Autodesk Inventor part; units mm, degrees
ref_plane "YZ Plane" through (0, 0, 0) normal (1, 0, 0) x (0, 1, 0)
ref_plane "XZ Plane" through (0, 0, 0) normal (0, 1, 0) x (-1, 0, 0)
ref_plane "XY Plane" through (0, 0, 0) normal (0, 0, 1) x (1, 0, 0)
sketch "Sketch1" plane through (0, 0, 0) normal (0, 1, 0) x (-1, 0, 0)
  circle A0 centre (0, 0) radius 9.525
  dimension "d0" = 19.05
extrude "Extrusion1" add sketch "Sketch1" along normal blind 5
sketch "Sketch2" plane through (0, 5, 0) normal (0, 1, 0) x (1, 0, 0)
  line L0 (0, 0) -> (0, 6.5)
  point P0 (-6.5, 0)
  point P1 (0, -6.5)
  point P2 (6.5, 0)
  dimension "d3" = 6.5
  dimension "d6" = 360
hole "Hole1" at (0, 5, -6.5) at (0, 5, 6.5) at (-6.5, 5, 0) at (6.5, 5, 0) direction (0, -1, 0) diameter 2.459 end through all
sketch "Sketch3" plane through (0, 5, 0) normal (0, 1, 0) x (1, 0, 0)
  circle A0 centre (0, 0) radius 2.1
  dimension "d15" = 4.2
extrude "Extrusion2" cut sketch "Sketch3" against normal through all
chamfer "Chamfer1" distance 0.25 angle 45 4 edges at (-2.1, 5, 0) (9.525, 5, 0) (9.525, 0, 0) (-2.1, 0, 0)
move or copy body "Move Body1" bodies to move or copy 1 copy no rotation origin (0, 0, 0) rotation axis (0, 1, 0) rotation angle 45
sketch "Sketch4" plane through (0, 0, 0) normal (1, 0, 0) x (0, 1, 0)
  line L0 (0, 0) -> (2.5, 0)
  dimension "d22" = 2.5
hole "Hole2" at (0, 2.5, 0) direction (1, 0, 0) diameter 2.459 end through all
properties part number "pololu-mounting-hub"
Build history of the part. All positions in model axes, mm. Round coordinates to 2 decimals unless told otherwise and drop trailing zeros. Order: outer loops, then holes, each group sorted by start corner. A loop starts at its lowest first (then second) coordinate and runs counter-clockwise, first axis right, second up. Notation, with made-up numbers: (-4.5, -15.75) -> (12.5, -15.75) arc R31 ccw to (12.5, 17.25) -> close; hole circle Ø11 at (85, 76). An arc over 180 degrees is marked (long way). Answer in a Markdown table with one row per item.
1) Mould opens along X. For faces 1 (the cylindrical face through (-4.028, 2.465, -3.506)), 2 (the cylindrical face through (6.433, 2.468, -7.025)), 3 (the cylindrical face through (5.668, 2.131, 1.173)) say: released by +X, released by -X, zero draft, split by the parting line, or undercut.
Values:
| item | result |
|---|---|
| face 1 | undercut |
| face 2 | split by the parting line |
| face 3 | zero draft |
2) Pin check, flat tip, straight feed: P1, Ø2, axis at y = 2.5, z = -5, coming from the +X side. Stop position of the tip, or through.
Values:
| item | result |
|---|---|
| P1 | x = 8.64 |
3) Band-saw the part on B-B on x = 0. Give the cut face in (y, z) (3 decimals), and give its area (3 significant figures).
Values:
| item | result |
|---|---|
| outline | (0, -9.275) -> (0.25, -9.525) -> (4.75, -9.525) -> (5, -9.275) -> (5, -2.35) -> (4.75, -2.1) -> (0.25, -2.1) -> (0, -2.35) -> close; (0, 2.35) -> (0.25, 2.1) -> (4.75, 2.1) -> (5, 2.35) -> (5, 9.275) -> (4.75, 9.525) -> (0.25, 9.525) -> (0, 9.275) -> close |
| area | 74.0 mm2 |
4) Wall check: L1, parallel to X at y = 0.85, z = 0 (3 decimals); L2, parallel to Z at x = 5.5, y = 1.65; L3, parallel to Z at x = 5, y = 4.35. Give the ranges that are in metal, low to high.
Values:
| item | result |
|---|---|
| L1 | -9.525 to -2.1, 2.1 to 9.525 |
| L2 | -7.78 to -5.43, -3.76 to -0.89, 0.89 to 3.76, 5.43 to 7.78 |
| L3 | -8.11 to -5.76, -3.43 to 3.43, 5.76 to 8.11 |
5) Band-saw the part on A-A on z = 0. Give the number of separate pieces and of enclosed holes in the cut face, and give its area (3 significant figures).
Values:
| item | result |
|---|---|
| separate pieces | 3 |
| enclosed holes | 0 |
| area | 55.7 mm2 |
